```python
from build123d import *

# Parameters (mm, degrees)
SKETCH1_W                = 30
SKETCH1_H                = 30
BOSS_EXTRUDE1_DEPTH      = 7
SKETCH2_W                = 7
SKETCH2_H                = 30
BOSS_EXTRUDE2_DEPTH      = 40
SKETCH3_W                = 30
SKETCH3_H                = 7.5
BOSS_EXTRUDE3_DEPTH      = 15
CUT_EXTRUDE1_DEPTH       = 2.5
M4_CLEARANCE_HOLE1_D     = 4.3
M4_CLEARANCE_HOLE1_DEPTH = 6
M4_CLEARANCE_HOLE1_TIP   = 1.291850331
CUT_EXTRUDE3_DEPTH       = 13


with BuildPart() as part:
    # Sketch1 → Boss-Extrude1 (new body)
    with BuildSketch(Plane(origin=(0, 0, 0), x_dir=(1, 0, 0), z_dir=(0, 1, 0))):
        Rectangle(SKETCH1_W, SKETCH1_H)
    extrude(amount=BOSS_EXTRUDE1_DEPTH)

    # Sketch2 → Boss-Extrude2 (add)
    with BuildSketch(Plane(origin=(0, 7, 0), x_dir=(1, 0, 0), z_dir=(0, 1, 0))):
        with Locations((11.5, 0)):
            Rectangle(SKETCH2_W, SKETCH2_H)
    extrude(amount=BOSS_EXTRUDE2_DEPTH)

    # Sketch3 → Boss-Extrude3 (add)
    with BuildSketch(Plane.ZY.offset(-8)):
        with Locations((0, 43.25)):
            Rectangle(SKETCH3_W, SKETCH3_H)
    extrude(amount=BOSS_EXTRUDE3_DEPTH)

    # Sketch4 → Cut-Extrude1 (cut)
    with BuildSketch(Plane.XZ.offset(-39.5)):
        Polygon((0.5, -4.330127019), (4.25, -2.165063509), (4.25, 2.165063509), (0.5, 4.330127019), (-3.25, 2.165063509), (-3.25, -2.165063509), align=None)
    extrude(amount=-CUT_EXTRUDE1_DEPTH, mode=Mode.SUBTRACT)

    # M4 Clearance Hole1
    with Locations(Plane(origin=(0, 47, 0), x_dir=(-1, 0, 0), z_dir=(0, 1, 0))):
        with Locations((-0.5, 0)):
            Hole(M4_CLEARANCE_HOLE1_D / 2, depth=M4_CLEARANCE_HOLE1_DEPTH)
            with Locations((0, 0, -(M4_CLEARANCE_HOLE1_DEPTH + M4_CLEARANCE_HOLE1_TIP / 2))):  # 118° drill point
                Cone(0, M4_CLEARANCE_HOLE1_D / 2, M4_CLEARANCE_HOLE1_TIP, mode=Mode.SUBTRACT)

    # Sketch8 → Cut-Extrude3 (cut)
    with BuildSketch(Plane(origin=(15, 0, 0), x_dir=(0, 0, -1), z_dir=(1, 0, 0))):
        with BuildLine():
            Line((-15, 10), (-15, 7))
            ThreePointArc((-15, 7), (-13.5, 8.5), (-15, 10))
        make_face()
        with BuildLine():
            Line((15, 10), (15, 7))
            ThreePointArc((15, 7), (13.5, 8.5), (15, 10))
        make_face()
    extrude(amount=-CUT_EXTRUDE3_DEPTH, mode=Mode.SUBTRACT)


solid = part.part
```
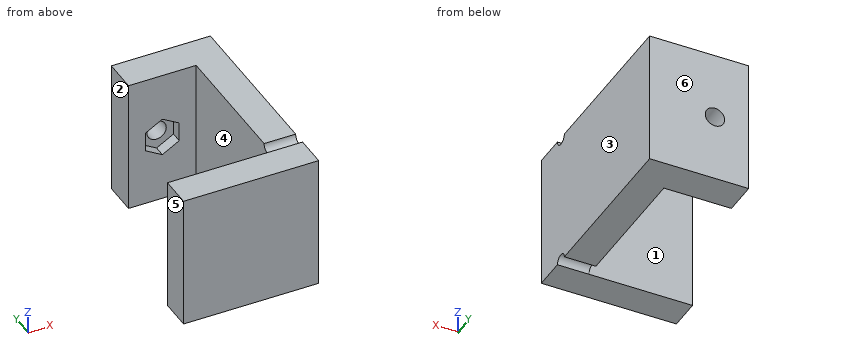
For this review, take the finished solid that the model builds, in its own axes (mm). Face numbers are marked on the shaded views. A direction names the side the tool comes from. Coordinates: 2 decimals unless noted, no trailing zeros. Loops run counter-clockwise (first coordinate to the right, second up) from the corner with the lowest first, then second, coordinate; pieces in that order, holes last.
1. Add section A-A, the plane z = 0. Give the boundary of the cut face in (x, y).
2. Add section B-B, the plane x = 3.5. Give the boundary of the cut face in (y, z).
3. Add section D-D, the plane y = 34. Give the boundary of the cut face in (x, z), then the cut area to 3 significant figures.
4. Add section C-C, the plane z = 5.5. Give the boundary of the cut face in (x, y), then the cut area to 4 significant figures.
5. For line 1 (Y direction, x = -2, z = -10.5); line 2 (Z direction, x = 0.5, y = 44.05); line 3 (X direction, y = 35, z = 10.5), list the stretches that pass through material, from the lowest coordinate up.
6. Insertion check: P1, Ø1, axis at y = 22.5, z = 6.5, coming from the -X side; P2, Ø2, axis at y = 42, z = 7, coming from the -X side; P3, Ø3.5, axis at x = 0.5, z = 0, coming from the +Y side. Each pin has a flat end and moves straight along its axis. Give the tip position at first contact, or say it passes through.
7. Mouldability with a two-part tool opening along Y and no side actions: class the marked faces 4, 5 and 6 as +Y half, -Y half, draft (parallel to the pull), parting line (faces both ways), or undercut.
8. For the marked faces 1, 2 and 3, list the 3-axis set-ups (+Z, -Z, +X, -X, +Y, -Y) from which the entire face can be reached by the end or side of a thin tool; tool diameter is ignored.
Result:
1. outline: (-15, 0) - (15, 0) - (15, 47) - (2.65, 47) - (2.65, 42) - (4.25, 42) - (4.25, 39.5) - (8, 39.5) - (8, 7) - (-15, 7) - close; (-7, 39.5) - (-3.25, 39.5) - (-3.25, 42) - (-1.65, 42) - (-1.65, 47) - (-7, 47) - close
2. outline: (0, -15) - (7, -15) - (7, 15) - (0, 15) - close; (39.5, -15) - (47, -15) - (47, 15) - (39.5, 15) - (39.5, 2.6) - (42, 2.6) - (42, -2.6) - (39.5, -2.6) - close
3. outline: (8, -15) - (15, -15) - (15, 15) - (8, 15) - close
3. area: 210 mm2
4. outline: (-15, 0) - (15, 0) - (15, 47) - (-7, 47) - (-7, 39.5) - (8, 39.5) - (8, 7) - (-15, 7) - close
4. area: 602.5 mm2
5. line 1: y = 0 to 7, 39.5 to 47
5. line 2: z = -15 to -2.15, 2.15 to 15
5. line 3: x = 8 to 15
6. P1: stops at x = 8
6. P2: stops at x = -7
6. P3: stops at y = 7
7. face 4: undercut
7. face 5: draft
7. face 6: +Y half
8. face 1: +Z, -Z, -X
8. face 2: +Z, -Z, -X, +Y
8. face 3: +Z, -Z, +X, +Y, -Y
